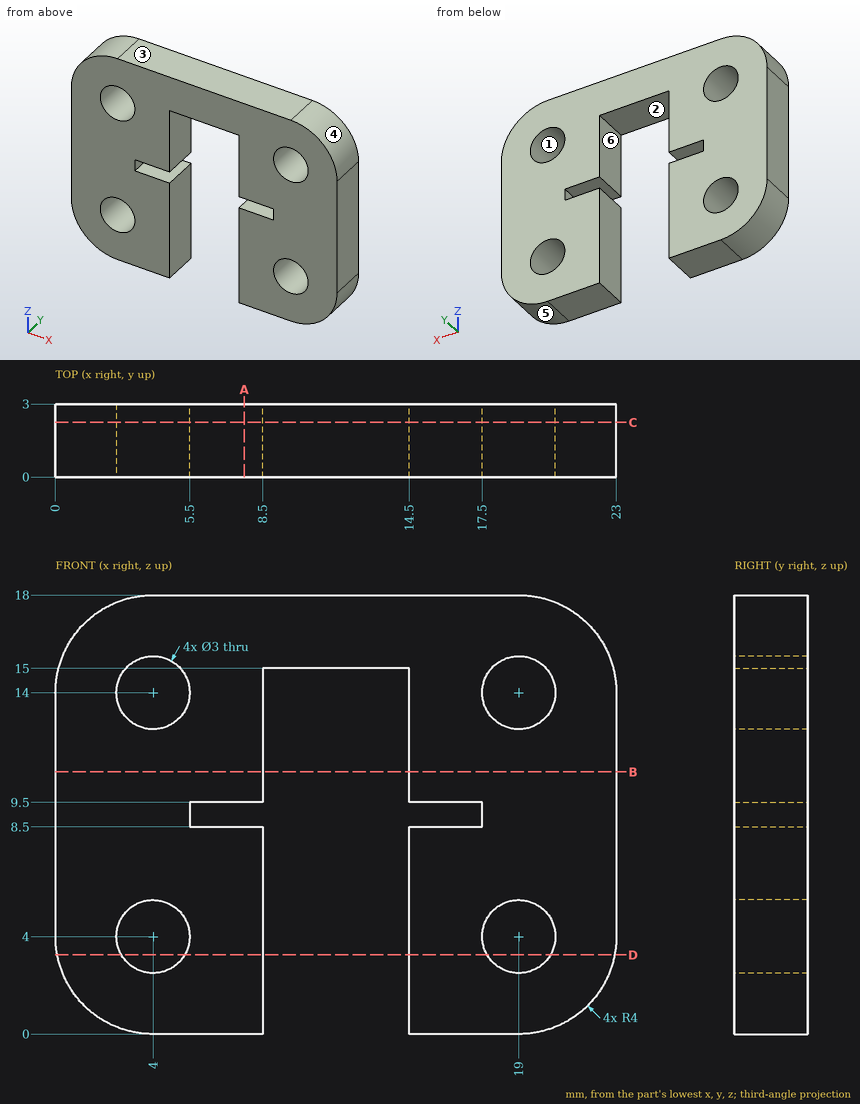
The drawing under review shows one solid part. Ordinate dimensions are in mm from its lowest x, y, z. A direction names the side the tool comes from. Coordinates: 2 decimals unless noted, no trailing zeros. Write each loop counter-clockwise with the first axis right and the second up, starting at its lowest first coordinate (ties: lowest second). Pieces come first, ordered by that corner, then holes. Notation, with made-up numbers: (-3, 10) -> (34, 10) arc R21 cw to (34, 26) -> close; hole circle Ø7 at (43.25, 85.25). An arc over 180 degrees is marked (long way). One line per item, written item: value. Start each with the question number.
Q1. Add section A-A, the plane x = 7.75. Give the boundary of the cut face in (y, z), then the cut area to 3 significant figures.
Q2. Add section B-B, the plane z = 10.75. Give the boundary of the cut face in (x, y), then the cut area to 3 significant figures.
Q3. Add section C-C, the plane y = 2.25. Give the boundary of the cut face in (x, z), then the cut area to 3 significant figures.
Q4. For the marked faces 5 and 6, list the 3-axis set-ups (+Z, -Z, +X, -X, +Y, -Y) from which the entire face can be reached by the end or side of a thin tool; tool diameter is ignored.
Q5. The part is to be moulded in two halves that separate along X. For the marked faces 1, 2, 3 and 4, say which applies: +X half, -X half, draft (parallel to the pull), parting line (faces both ways), or undercut.
Q6. To check wall thickness, follow probe 1 along Z at (x, y) = (17.75, 0.8); probe 2 along Z at (x, y) = (4.25, 1); probe 3 along X at (y, z) = (1.4, 13.25). State the ranges of each line that lie inside material, in increasing order.
Q7. Clearance check with flat-ended pins moving along their axes: P1, Ø0.9, axis at x = 12.5, y = 1.5, coming from the -Z side; P2, Ø0.9, axis at y = 1, z = 3, coming from the -X side. State where each tip first meets the part, or that it passes through.
Q8. Add section D-D, the plane z = 3.25. Give the boundary of the cut face in (x, y), then the cut area to 3 significant figures.
Response:
1. outline: (0, 0) -> (3, 0) -> (3, 8.5) -> (0, 8.5) -> close; (0, 9.5) -> (3, 9.5) -> (3, 18) -> (0, 18) -> close
1. area: 51.0 mm²
2. outline: (0, 0) -> (8.5, 0) -> (8.5, 3) -> (0, 3) -> close; (14.5, 0) -> (23, 0) -> (23, 3) -> (14.5, 3) -> close
2. area: 51.0 mm²
3. outline: (0, 4) arc R4 ccw to (4, 0) -> (8.5, 0) -> (8.5, 8.5) -> (5.5, 8.5) -> (5.5, 9.5) -> (8.5, 9.5) -> (8.5, 15) -> (14.5, 15) -> (14.5, 9.5) -> (17.5, 9.5) -> (17.5, 8.5) -> (14.5, 8.5) -> (14.5, 0) -> (19, 0) arc R4 ccw to (23, 4) -> (23, 14) arc R4 ccw to (19, 18) -> (4, 18) arc R4 ccw to (0, 14) -> close; hole circle Ø3 at (4, 4); hole circle Ø3 at (4, 14); hole circle Ø3 at (19, 4); hole circle Ø3 at (19, 14)
3. area: 276 mm²
4. face 5: -Z, +X, +Y, -Y
4. face 6: -Z, +Y, -Y
5. face 1: undercut
5. face 2: undercut
5. face 3: draft
5. face 4: +X half
6. probe 1: 0 to 3.17, 4.83 to 13.17, 14.83 to 18
6. probe 2: 0 to 2.52, 5.48 to 12.52, 15.48 to 18
6. probe 3: 0 to 2.7, 5.3 to 8.5, 14.5 to 17.7, 20.3 to 23
7. P1: z = 15
7. P2: x = 0.04
8. outline: (0.07, 0) -> (2.7, 0) -> (2.7, 3) -> (0.07, 3) -> close; (5.3, 0) -> (8.5, 0) -> (8.5, 3) -> (5.3, 3) -> close; (14.5, 0) -> (17.7, 0) -> (17.7, 3) -> (14.5, 3) -> close; (20.3, 0) -> (22.93, 0) -> (22.93, 3) -> (20.3, 3) -> close
8. area: 35.0 mm²
